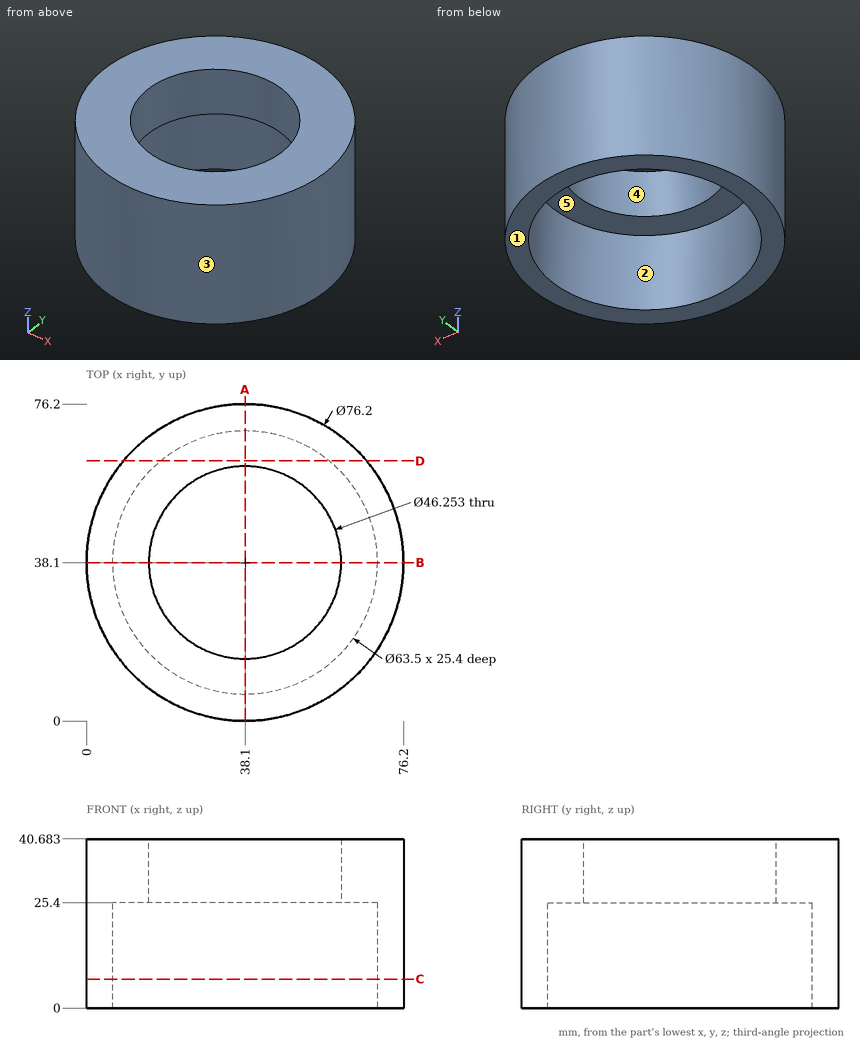
Input: dimensioned drawing with shaded views. Units: mm. Origin: part minimum x, y, z. A direction names the side the tool comes from. Coordinates: 2 decimals unless noted, no trailing zeros. Loops run counter-clockwise (first coordinate to the right, second up) from the corner with the lowest first, then second, coordinate; pieces in that order, holes last. Notation, with made-up numbers: M -14.75,-37 L 13.25,-37 A15 cw 13.25,-24 Z; hole C 66,68 d5. An arc over 180 degrees is marked long. Put each result on its own line as item: value.
(1) Cut plane A-A on x = 38.1. Return the cut outline in (y, z), then the cut area to 3 significant figures.
Answer sheet:
outline: M 0,0 L 6.35,0 L 6.35,25.4 L 14.97,25.4 L 14.97,40.68 L 0,40.68 Z; M 61.23,25.4 L 69.85,25.4 L 69.85,0 L 76.2,0 L 76.2,40.68 L 61.23,40.68 Z
area: 780 mm^2
(2) Draft query along X for the marked faces 1, 2 and 3. Return one class per face: pulls with the +X half, pulls with the -X half, needs draft (parallel to the pull), parting line crosses it, or undercut.
Answer sheet:
face 1: needs draft
face 2: undercut
face 3: parting line crosses it
(3) Cut plane C-C on z = 7. Return the cut outline in (x, y), then the cut area to 3 significant figures.
Answer sheet:
outline: C 38.1,38.1 d76.2; hole C 38.1,38.1 d63.5
area: 1,390 mm^2
(4) Cut plane D-D on y = 62.5. Return the cut outline in (x, z) (1 decimal), then the cut area to 3 significant figures.
Answer sheet:
outline: M 8.8,0 L 17.8,0 L 17.8,25.4 L 58.4,25.4 L 58.4,0 L 67.4,0 L 67.4,40.7 L 8.8,40.7 Z
area: 1,350 mm^2
(5) Material intervals for probe 1 along X at (y, z) = (39, 16.5); probe 2 along Y at (x, z) = (38.1, 32.25); probe 3 along Z at (x, y) = (13, 24), sorted ascending.
Answer sheet:
probe 1: x = 0.01 to 6.36, 69.84 to 76.19
probe 2: y = 0 to 14.97, 61.23 to 76.2
probe 3: z = 25.4 to 40.68
(6) First-contact query: pin 1 (2 mm diameter, centred on y = 31.5, z = 18.5, fed in from -X); pin 2 (2 mm diameter, centred on y = 41.5, z = 26.5, fed in from -X); pin 3 (1 mm diameter, centred on x = 22, z = 14.5, fed in from +Y). Flat tips, straight axial feed; report the tip coordinate or a pass-through.
Answer sheet:
pin 1: stops at x = 0.41
pin 2: stops at x = 0.08
pin 3: stops at y = 72.86
(7) Access query for the marked faces 4 and 5. Directions: +Z, -Z, +X, -X, +Y, -Y. A direction counts if a zero-diameter tool reaches every point of the face in a straight line with its end or side. Return the directions, or none.
Answer sheet:
face 4: +Z, -Z
face 5: -Z
